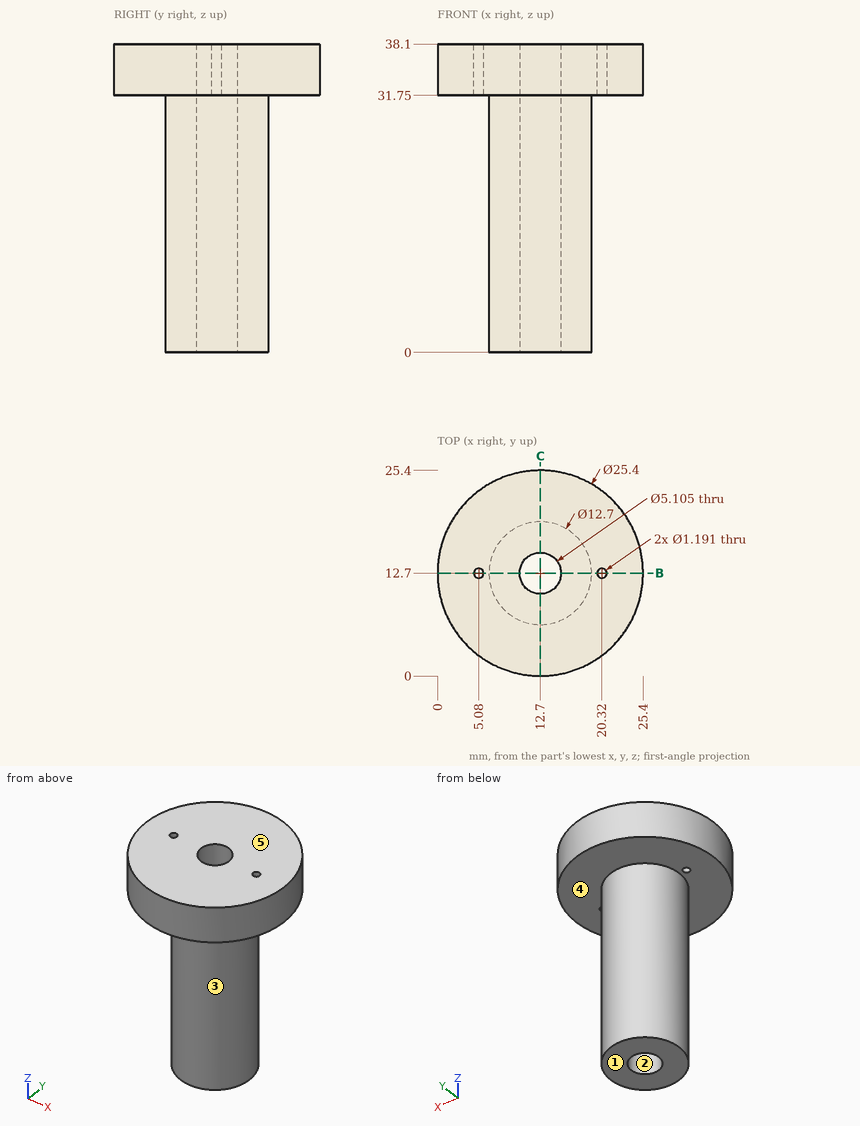
Can you work these out from the drawing? Everything is in mm from the part's minimum corner. A direction names the side the tool comes from. Coordinates: 2 decimals unless noted, no trailing zeros. Write each loop counter-clockwise with the first axis right and the second up, starting at its lowest first coordinate (ties: lowest second). Pieces come first, ordered by that corner, then holes. Notation, with made-up numbers: (30.25, 56) -> (76.25, 56) arc R17 cw to (76.25, 72) -> close; hole circle Ø2 at (74.25, 41.25). An arc over 180 degrees is marked (long way). Write each question's results on one line, items separated by ' | '. Start each with the question number.
Item 1: If we section it at C-C, the plane x = 12.7: Write out the boundary of the cut face in (y, z).
Item 2: Thinking about a two-plate mould opening in Y: for the marked faces 1, 2 and 3, which applies, released by +Y, released by -Y, zero draft, split by the parting line, or undercut?
Item 3: On a 3-axis mill with a long thin cutter (end or side, diameter ignored), from which of +Z, -Z, +X, -X, +Y, -Y can I reach the whole of each face in a straight line? I mean the marked faces 4 and 5. Say none if no direction works.
Item 4: I'm going to push flat-ended pins straight in: P1, Ø1.5, axis at x = 20.32, y = 12.7, coming from the -Z side; P2, Ø4, axis at y = 13.5, z = 25.5, coming from the -X side; P3, Ø10, axis at x = 15, z = 23, coming from the +Y side; P4, Ø10, axis at x = 21, y = 15.5, coming from the -Z side. Where does each tip first touch, or does it pass through?
Item 5: If we section it at B-B, the plane y = 12.7: Count the separate pieces of the cut face and the enclosed holes in it, and give its area (3 significant figures).
Item 6: Please list where these lines run through material, in increasing order: probe 1 along Y at (x, z) = (12.7, 13); probe 2 along Z at (x, y) = (14.5, 5.5); probe 3 along Y at (x, z) = (20.32, 34.25) (1 decimal).
Answer block:
1) outline: (0, 31.75) -> (6.35, 31.75) -> (6.35, 0) -> (10.15, 0) -> (10.15, 38.1) -> (0, 38.1) -> close; (15.25, 0) -> (19.05, 0) -> (19.05, 31.75) -> (25.4, 31.75) -> (25.4, 38.1) -> (15.25, 38.1) -> close
2) face 1: zero draft | face 2: undercut | face 3: split by the parting line
3) face 4: -Z | face 5: +Z, +X, -X, +Y, -Y
4) P1: z = 31.75 | P2: x = 6.35 | P3: y = 19.05 | P4: z = 0
5) separate pieces: 4 | enclosed holes: 0 | area: 355 mm²
6) probe 1: 6.35 to 10.15, 15.25 to 19.05 | probe 2: 31.75 to 38.1 | probe 3: 2.5 to 12.1, 13.3 to 22.9
